Autodesk Inventor part; units mm, degrees
ref_plane "YZ Plane" through (0, 0, 0) normal (1, 0, 0) x (0, 1, 0)
ref_plane "XZ Plane" through (0, 0, 0) normal (0, 1, 0) x (-1, 0, 0)
ref_plane "XY Plane" through (0, 0, 0) normal (0, 0, 1) x (1, 0, 0)
sketch "Sketch1" plane through (0, 0, 0) normal (1, 0, 0) x (0, 1, 0)
  line L0 (7.1501, 0) -> (13.4874, 0)
  line L1 (20.6375, -7.1501) -> (20.6375, -7.1501)
  line L2 (13.4874, -14.3002) -> (7.1501, -14.3002)
  line L3 (0, -7.1501) -> (0, -7.1501)
  arc A0 (20.6375, -7.1501) -> (13.4874, 0) centre (13.4874, -7.1501) ccw
  arc A1 (13.4874, -14.3002) -> (20.6375, -7.1501) centre (13.4874, -7.1501) ccw
  arc A2 (0, -7.1501) -> (7.1501, -14.3002) centre (7.1501, -7.1501) ccw
  arc A3 (7.1501, 0) -> (0, -7.1501) centre (7.1501, -7.1501) ccw
  point P0 (0, 0)
  point P1 (20.6375, -14.3002)
  point P2 (20.6375, 0)
  point P3 (0, -14.3002)
  dimension "d0" = 20.6375
  dimension "d1" = 14.3002
  dimension "d2" = 7.1501
extrude "Extrusion1" add sketch "Sketch1" along normal blind 3.175
sketch "Sketch2" plane through (3.175, 0, 0) normal (1, 0, 0) x (0, 0, -1)
  line L0 (0, 13.4874) -> (0, 7.1501)
  line L1 (0, 10.3187) -> (14.3002, 10.3187)
  line L2 (14.3002, 7.1501) -> (14.3002, 13.4874)
  arc A0 (14.3002, 13.4874) -> (0, 13.4874) centre (7.1501, 13.4874) ccw
  arc A1 (0, 7.1501) -> (14.3002, 7.1501) centre (7.1501, 7.1501) ccw
  line L3 (7.1501, 13.4874) -> (7.1501, 7.1501)
  circle A2 centre (7.1501, 10.3187) radius 3.1686
  point P0 (0, 0)
extrude "Extrusion2" add sketch "Sketch2" along normal blind 63.5 contours A2 L3 L1 | L1 L3 A2 | L3 A2 L1 | L1 A2 L3
thread "Thread1"
fillet "Fillet1" radius 0.508 8 edges at (3.175, 10.3187, 0) (3.175, 0, -7.1501) (3.175, 10.3187, -14.3002) (3.175, 20.6375, -7.1501) (0, 10.3187, 0) (0, 0, -7.1501) (0, 10.3187, -14.3002) (0, 20.6375, -7.1501)
properties part number "TeeBolt"
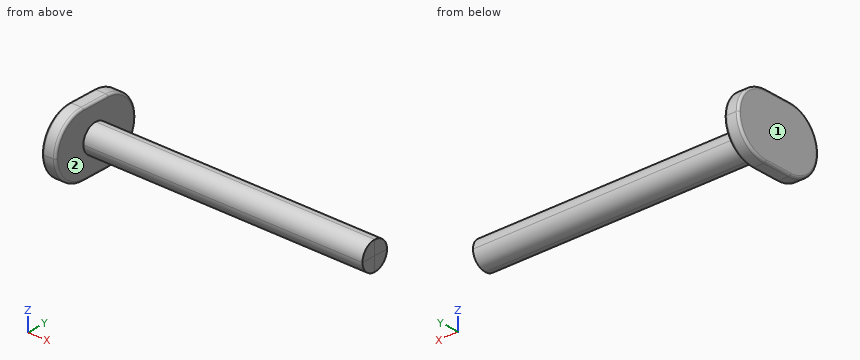
Part model, mm, in its own coordinate system. Face numbers are marked on the shaded views. A direction names the side the tool comes from. Give positions to 0.01 mm unless a question says otherwise; leave off trailing zeros. Write each loop counter-clockwise with the first axis right and the second up, starting at its lowest first coordinate (ties: lowest second). Pieces come first, ordered by that corner, then holes.
1) Which spindle directions (+Z, -Z, +X, -X, +Y, -Y) get a long thin tool onto all of the face, cutting with end or side? Do the marked faces 1 and 2. Say none if no direction does.
Resolved:
face 1: +Z, -Z, -X, +Y, -Y
face 2: +X
2) Pin check, flat tips, straight feed: pin 1 (6 mm diameter, centred on x = 34, y = 5, fed in from +Z); pin 2 (12 mm diameter, centred on x = 12.5, y = 9.5, fed in from +Z); pin 3 (1 mm diameter, centred on y = 6, z = -9.5, fed in from -X); pin 4 (5 mm diameter, centred on y = 2.5, z = -6, fed in from +X) (3 decimals). Stop position of each tip, or through.
Resolved:
pin 1: stops at z = -4.99
pin 2: stops at z = -3.98
pin 3: stops at x = 0
pin 4: stops at x = 3.175
3) Cut at A-A on y = 8.25. Write the cut outline in (x, z) (3 decimals), then the cut area to 3 significant figures.
Resolved:
outline: (0, -13.792) arc R0.508 ccw to (0.508, -14.3) - (2.667, -14.3) arc R0.508 ccw to (3.175, -13.792) - (3.175, -9.55) - (66.675, -9.55) - (66.675, -4.75) - (3.175, -4.75) - (3.175, -0.508) arc R0.508 ccw to (2.667, 0) - (0.508, 0) arc R0.508 ccw to (0, -0.508) - close
area: 350 mm2
4) Probe L1, parallel to X at y = 5.25, z = -4.25 (3 decimals); L2, parallel to Y at x = 6, z = -7; L3, parallel to Y at x = 45, z = -5. List the from-to ranges inside material, lowest first.
Resolved:
L1: x = 0 to 3.175
L2: y = 7.15 to 13.48
L3: y = 7.99 to 12.65
5) Cut at B-B on x = 8.5. Write the cut outline in (y, z).
Resolved:
outline: circle Ø6.34 at (10.32, -7.15)
6) Cut at C-C on y = 12.25. Write the cut outline in (x, z) (3 decimals).
Resolved:
outline: (0, -13.792) arc R0.508 ccw to (0.508, -14.3) - (2.667, -14.3) arc R0.508 ccw to (3.175, -13.792) - (3.175, -9.662) - (66.675, -9.662) - (66.675, -4.638) - (3.175, -4.638) - (3.175, -0.508) arc R0.508 ccw to (2.667, 0) - (0.508, 0) arc R0.508 ccw to (0, -0.508) - close
